Could you check a few things on this model? Use its own coordinates, in mm. A direction names the side the tool comes from. Coordinates: 2 decimals unless noted, no trailing zeros. Order: outer loops, then holes, each group sorted by start corner. A loop starts at its lowest first (then second) coordinate and runs counter-clockwise, first axis right, second up.
```python
from build123d import *

# Parameters (mm, degrees)
BOSS_EXTRUDE2_DEPTH = 60
CUT_EXTRUDE2_DEPTH  = 123.065556157


with BuildPart() as part:
    # Sketch1 → Boss-Extrude2 (new, symmetric)
    with BuildSketch(Plane(origin=(0, 0, 0), x_dir=(1, 0, 0), z_dir=(0, 1, 0))):
        with BuildLine():
            Line((15, -10), (-15, -10))
            ThreePointArc((-15, -10), (-18.535533906, -8.535533906), (-20, -5))
            Line((-20, -5), (-20, 5))
            ThreePointArc((-20, 5), (-18.535533906, 8.535533906), (-15, 10))
            Line((-15, 10), (15, 10))
            ThreePointArc((15, 10), (18.535533906, 8.535533906), (20, 5))
            Line((20, 5), (20, -5))
            ThreePointArc((20, -5), (18.535533906, -8.535533906), (15, -10))
        make_face()
    extrude(amount=BOSS_EXTRUDE2_DEPTH, both=True)

    # Sketch3 → Cut-Extrude2 (cut, through all)
    with BuildSketch(Plane(origin=(0, 60, 0), x_dir=(1, 0, 0), z_dir=(0, 1, 0))):
        with BuildLine():
            Line((12.5, -7.5), (-12.5, -7.5))
            ThreePointArc((-12.5, -7.5), (-16.035533906, -6.035533906), (-17.5, -2.5))
            Line((-17.5, -2.5), (-17.5, 2.5))
            ThreePointArc((-17.5, 2.5), (-16.035533906, 6.035533906), (-12.5, 7.5))
            Line((-12.5, 7.5), (12.5, 7.5))
            ThreePointArc((12.5, 7.5), (16.035533906, 6.035533906), (17.5, 2.5))
            Line((17.5, 2.5), (17.5, -2.5))
            ThreePointArc((17.5, -2.5), (16.035533906, -6.035533906), (12.5, -7.5))
        make_face()
    extrude(amount=-CUT_EXTRUDE2_DEPTH, mode=Mode.SUBTRACT)


solid = part.part
```
Item 1: I need wall thicknesses on line 1 (Z direction, x = -0.5, y = -37); line 2 (X direction, y = 35.5, z = -3); line 3 (X direction, y = -11.5, z = 7). Which ranges of each line are inside material? Lowest first, please.
Item 2: Suppose I cut it at C-C (y = 31.5). List the corners of the cut face in (x, z) for me.
Item 3: Thinking about a two-plate mould opening in X: for faces 3 (the face through (16, 0.84, -6.07)), 4 (the face through (-20, 1, 0)), 5 (the face through (3, 60, 8)), 6 (the face through (19, 1, 8)), which applies, +X half, -X half, draft (parallel to the pull), parting line (faces both ways), or undercut?
Item 4: Suppose I cut it at B-B (z = 0.25). List the corners of the cut face in (x, y) for me, and give its area (3 significant figures).
Item 5: Which directions (+Z, -Z, +X, -X, +Y, -Y) give clear straight access to the entire face, cutting with the end or side of a thin tool? Please do faces 1 (the face through (0, 1, 7.5)), 2 (the face through (3, -60, 8)).
Item 6: Suppose I cut it at A-A (x = 11). List the corners of the cut face in (y, z) for me.
Item 7: For pin 1 Ø2 at (y, z) = (30.5, -5.5) entering from -X, with a flat end and sliding along its axis, tell me the tip position at first contact or that it passes through.
Geometry results:
1. line 1: z = -10 to -7.5, 7.5 to 10
1. line 2: x = -20 to -17.47, 17.47 to 20
1. line 3: x = -19.58 to -14.68, 14.68 to 19.58
2. outline: (-20, -5) arc R5 ccw to (-15, -10) - (15, -10) arc R5 ccw to (20, -5) - (20, 5) arc R5 ccw to (15, 10) - (-15, 10) arc R5 ccw to (-20, 5) - close; hole (-17.5, -2.5) arc R5 ccw to (-12.5, -7.5) - (12.5, -7.5) arc R5 ccw to (17.5, -2.5) - (17.5, 2.5) arc R5 ccw to (12.5, 7.5) - (-12.5, 7.5) arc R5 ccw to (-17.5, 2.5) - close
3. face 3: undercut
3. face 4: -X half
3. face 5: draft
3. face 6: +X half
4. outline: (-20, -60) - (-17.5, -60) - (-17.5, 60) - (-20, 60) - close; (17.5, -60) - (20, -60) - (20, 60) - (17.5, 60) - close
4. area: 600 mm2
5. face 1: +Y, -Y
5. face 2: +Z, -Z, +X, -X, -Y
6. outline: (-60, -10) - (60, -10) - (60, -7.5) - (-60, -7.5) - close; (-60, 7.5) - (60, 7.5) - (60, 10) - (-60, 10) - close
7. pin 1: stops at x = -20
